Print and shaded views of the part. All mm, measured from the part's lowest x, y and z. Round coordinates to 2 decimals unless told otherwise and drop trailing zeros. Loops run counter-clockwise (first coordinate to the right, second up) from the corner with the lowest first, then second, coordinate; pieces in that order, holes last. Notation, with made-up numbers: (20, 87) - (76, 87) arc R34 ccw to (76, 124) - close; hole circle Ø2 at (27.25, 75). An arc over 180 degrees is marked (long way). Answer as a JSON object with one key per item and string values.
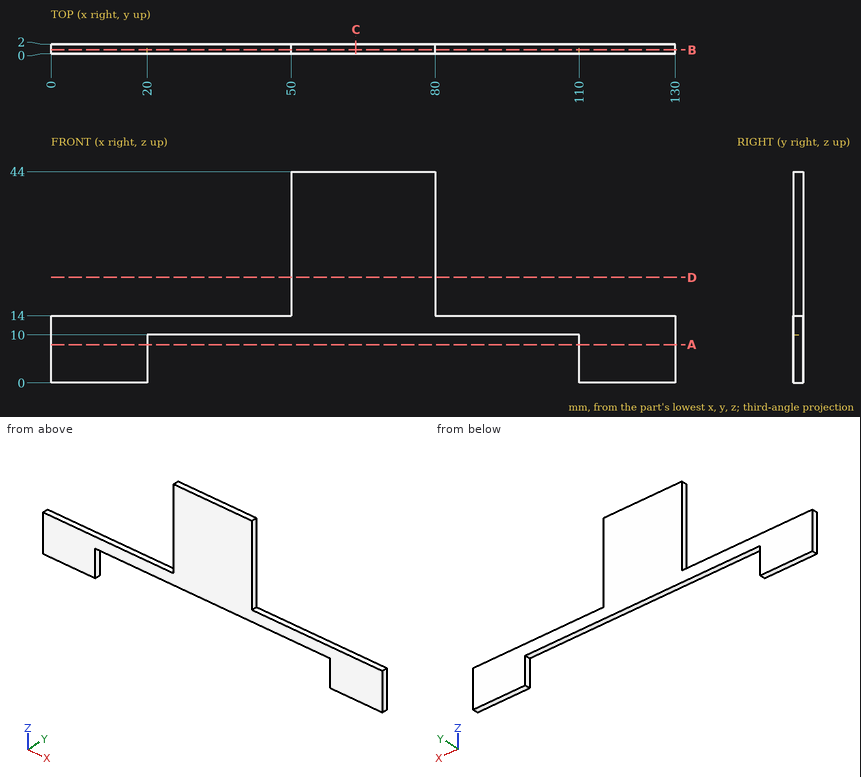
1) Slice it at A-A on z = 8. List the corners of the cut face in (x, y), then the cut area to 3 significant figures.
Values follow:
{"outline": "(0, 0) - (20, 0) - (20, 2) - (0, 2) - close; (110, 0) - (130, 0) - (130, 2) - (110, 2) - close", "area": "80.0 mm²"}
2) Slice it at C-C on x = 63.5. List the corners of the cut face in (y, z), then the cut area to 3 significant figures.
Values follow:
{"outline": "(0, 10) - (2, 10) - (2, 44) - (0, 44) - close", "area": "68.0 mm²"}
3) Slice it at B-B on y = 0.8. List the corners of the cut face in (x, z).
Values follow:
{"outline": "(0, 0) - (20, 0) - (20, 10) - (110, 10) - (110, 0) - (130, 0) - (130, 14) - (80, 14) - (80, 44) - (50, 44) - (50, 14) - (0, 14) - close"}
4) Drop flat-ended pins along their axis: P1, Ø1, axis at x = 108, y = 0.5, coming from the +Z side; P2, Ø1.5, axis at x = 48.5, z = 10, coming from the -Y side; P3, Ø1, axis at y = 0.5, z = 22, coming from the +X side. Give the stop position or say it passes through.
Values follow:
{"P1": "z = 14", "P2": "y = 0", "P3": "x = 80"}
5) Probe probe 1 along X at (y, z) = (1.7, 8); probe 2 along Z at (x, y) = (64.5, 1.15); probe 3 along Z at (x, y) = (14, 1.5). List the from-to ranges inside material, lowest first.
Values follow:
{"probe 1": "0 to 20, 110 to 130", "probe 2": "10 to 44", "probe 3": "0 to 14"}
6) Slice it at D-D on z = 22. List the corners of the cut face in (x, y), then the cut area to 3 significant figures.
Values follow:
{"outline": "(50, 0) - (80, 0) - (80, 2) - (50, 2) - close", "area": "60.0 mm²"}
